```python
from build123d import *

# Parameters (mm, degrees)
SKETCH2_W           = 8.65
SKETCH2_H           = 8.65
BOSS_EXTRUDE1_DEPTH = 7.2
FILLET1_R           = 2


with BuildPart() as part:
    # Sketch2 → Boss-Extrude1 (new body)
    with BuildSketch(Plane(origin=(0, 0, 0), x_dir=(1, 0, 0), z_dir=(0, 1, 0))):
        with Locations((4.325, 4.325)):
            Rectangle(SKETCH2_W, SKETCH2_H)
    extrude(amount=BOSS_EXTRUDE1_DEPTH)

    # Fillet1
    fillet1_edges = [part.edges().sort_by_distance(p)[0] for p in [
        (0, 3.6, -8.65),
    ]]
    fillet(fillet1_edges, radius=FILLET1_R)


solid = part.part
```
Could you check a few things on this model? Use its own coordinates, in mm. Round coordinates to 2 decimals unless told otherwise and drop trailing zeros. Loops run counter-clockwise (first coordinate to the right, second up) from the corner with the lowest first, then second, coordinate; pieces in that order, holes last. Notation, with made-up numbers: M 23,10.25 L 57,10.25 A10 ccw 57,26.25 Z; hole C 25,11.5 d9. An arc over 180 degrees is marked long. Write item = value, one per line.
1. I need wall thicknesses on probe 1 along X at (y, z) = (6, -6.75); probe 2 along X at (y, z) = (5.5, -7.5); probe 3 along Z at (x, y) = (1, 1.5). Which ranges of each line are inside material? Lowest first, please.
Results below:
probe_1 = 0 to 8.65
probe_2 = 0.19 to 8.65
probe_3 = -8.38 to 0
2. Thinking about a two-plate mould opening in Z: for faces 1 (the face through (5, 4, -8.65)), 2 (the face through (4, 7.2, -4)), 3 (the face through (4, 4, 0)), which applies, +Z half, -Z half, draft (parallel to the pull), parting line (faces both ways), or undercut?
Results below:
face_1 = -Z half
face_2 = draft
face_3 = +Z half
3. I want a section at A-A, the plane x = 1.25. Write out the boundary of the cut face in (y, z).
Results below:
outline = M 0,-8.5 L 7.2,-8.5 L 7.2,0 L 0,0 Z
